Part model, mm, in its own coordinate system. Coordinates: 2 decimals unless noted, no trailing zeros. Write each loop counter-clockwise with the first axis right and the second up, starting at its lowest first coordinate (ties: lowest second). Pieces come first, ordered by that corner, then holes. Notation, with made-up numbers: M 53.25,-9 L 61.25,-9 A29 ccw 61.25,14 Z; hole C 76,-11.5 d7. An arc over 180 degrees is marked long. Use a Markdown table: item, result. Add a question column.
Q1. Slice it at A-A on y = -9.5. Write the cut outline in (x, z), then the cut area to 3 significant figures.
Q2. Wall check: L1, parallel to Y at x = 55, z = 3.8; L2, parallel to X at y = -13, z = 1.5; L3, parallel to Y at x = -56.5, z = 1. Give the ranges that are in metal, low to high. Write a range as from..to.
Q3. Slice it at B-B on x = 55. Write the cut outline in (y, z).
Q4. Slice it at D-D on x = -66. Write the cut outline in (y, z), then the cut area to 3 significant figures.
Q5. Slice it at C-C on z = 7.25. Write the cut outline in (x, y), then the cut area to 3 significant figures.
from build123d import *

# Parameters (mm, degrees)
SKETCH1_W                               = 250
SKETCH1_H                               = 99
BOSS_EXTRUDE1_DEPTH                     = 10
CBORE_FOR_M5_HEX_HEAD_BOLT1_D           = 33
CBORE_FOR_M5_HEX_HEAD_BOLT1_CBORE_D     = 35
CBORE_FOR_M5_HEX_HEAD_BOLT1_CBORE_DEPTH = 5


with BuildPart() as part:
    # Sketch1 → Boss-Extrude1 (new body)
    with BuildSketch(Plane.XY):
        Rectangle(SKETCH1_W, SKETCH1_H)
    extrude(amount=BOSS_EXTRUDE1_DEPTH)

    # CBORE for M5 Hex Head Bolt1 (through all)
    with Locations(Plane(origin=(0, 0, 0), x_dir=(-1, 0, 0), z_dir=(0, 0, -1))):
        with Locations((-55, -9.5)):
            cbore_for_m5_hex_head_bolt1 = CounterBoreHole(CBORE_FOR_M5_HEX_HEAD_BOLT1_D / 2, CBORE_FOR_M5_HEX_HEAD_BOLT1_CBORE_D / 2, CBORE_FOR_M5_HEX_HEAD_BOLT1_CBORE_DEPTH)

    # Mirror1: CBORE for M5 Hex Head Bolt1 across plane
    add(cbore_for_m5_hex_head_bolt1.mirror(Plane(origin=(0, 0, 0), x_dir=(0, 0, 1), z_dir=(1, 0, 0))), mode=Mode.SUBTRACT)


solid = part.part
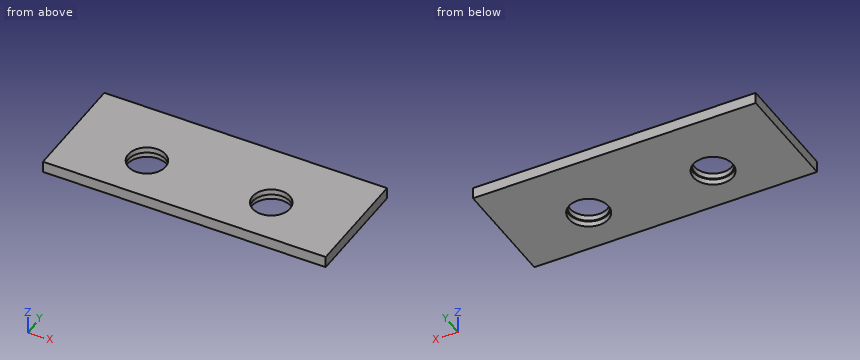
Recorded:
| question | item | result |
|---|---|---|
| 1 | outline | M -125,0 L -72.5,0 L -72.5,5 L -71.5,5 L -71.5,10 L -125,10 Z; M -38.5,5 L -37.5,5 L -37.5,0 L 37.5,0 L 37.5,5 L 38.5,5 L 38.5,10 L -38.5,10 Z; M 71.5,5 L 72.5,5 L 72.5,0 L 125,0 L 125,10 L 71.5,10 Z |
| 1 | area | 1,820 mm² |
| 2 | L1 | -49.5..-27, 8..49.5 |
| 2 | L2 | -125..-72.15, -37.85..37.85, 72.15..125 |
| 2 | L3 | -49.5..-26.94, 7.94..49.5 |
| 3 | outline | M -49.5,0 L -27,0 L -27,5 L -26,5 L -26,10 L -49.5,10 Z; M 7,5 L 8,5 L 8,0 L 49.5,0 L 49.5,10 L 7,10 Z |
| 4 | outline | M -49.5,0 L -23.11,0 L -23.11,5 L -21.8,5 L -21.8,10 L -49.5,10 Z; M 2.8,5 L 4.11,5 L 4.11,0 L 49.5,0 L 49.5,10 L 2.8,10 Z |
| 4 | area | 731 mm² |
| 5 | outline | M -125,-49.5 L 125,-49.5 L 125,49.5 L -125,49.5 Z; hole C -55,-9.5 d33; hole C 55,-9.5 d33 |
| 5 | area | 23,000 mm² |
